For this review, take the finished solid that the model builds, in its own axes (mm). A direction names the side the tool comes from. Coordinates: 2 decimals unless noted, no trailing zeros. Loops run counter-clockwise (first coordinate to the right, second up) from the corner with the lowest first, then second, coordinate; pieces in that order, holes last.
1. Take a section at B-B, the plane z = 0. State the section outline as (x, y) points.
2. Machinability: for faces 1 (the face through (8.8, -1.6, -2.3)), 2 (the face through (10, 0, -2.05)), 3 (the face through (19, 0, 0)), which of the approach directions +Z, -Z, +X, -X, +Y, -Y give a long, thin tool a straight path to every point of the face, cutting with its end or side? Answer none if there is none.
3. Clearance check with a flat-ended pin moving along its axis: P1, Ø5, axis at x = 7, z = 4, coming from the -Y side. State where the tip first meets the part, or that it passes through.
4. To check wall thickness, follow probe 1 along Z at (x, y) = (12.25, 1.15); probe 2 along Y at (x, z) = (7, -2.25); probe 3 along Y at (x, z) = (1, 3.5). State the ranges of each line that lie inside material, in increasing order.
5. Take a section at A-A, the plane x = 11.75. State the section outline as (y, z) points, then the cut area to 3 significant figures.
6. Take a section at C-C, the plane y = 1.55. State the section outline as (x, z) points, then the cut area to 3 significant figures.
7. Take a section at D-D, the plane z = -3. State the section outline as (x, y) points.
```python
from build123d import *

# Parameters (mm, degrees)
SKETCH1_W           = 19
SKETCH1_H           = 10
BOSS_EXTRUDE1_DEPTH = 2
CHAMFER2_SIZE       = 1
SKETCH2_W           = 17.6
SKETCH2_H           = 10
CUT_EXTRUDE4_DEPTH  = 0.4
CUT_EXTRUDE5_DEPTH  = 21.049937656
CHAMFER4_SIZE       = 3.5
CHAMFER4_SIZE2      = 2.450726384
CHAMFER5_SIZE       = 0.25


with BuildPart() as part:
    # Sketch1 → Boss-Extrude1 (new, symmetric)
    with BuildSketch(Plane(origin=(0, 0, 0), x_dir=(1, 0, 0), z_dir=(0, 1, 0))):
        with Locations((9.5, 0)):
            Rectangle(SKETCH1_W, SKETCH1_H)
        with BuildLine():
            Line((8.5, 2.05), (12.5, 2.05))
            ThreePointArc((12.5, 2.05), (14.55, 0), (12.5, -2.05))
            Line((12.5, -2.05), (8.5, -2.05))
            ThreePointArc((8.5, -2.05), (6.45, 0), (8.5, 2.05))
        make_face(mode=Mode.SUBTRACT)
    extrude(amount=BOSS_EXTRUDE1_DEPTH, both=True)

    # Chamfer2
    chamfer2_edges = [part.edges().sort_by_distance(p)[0] for p in [
        (19, 0, -5),
        (19, 0, 5),
    ]]
    chamfer(chamfer2_edges, length=CHAMFER2_SIZE)

    # Sketch2 → Cut-Extrude4 (cut)
    with BuildSketch(Plane(origin=(0, -2, 0), x_dir=(1, 0, 0), z_dir=(0, 1, 0))):
        with Locations((8.8, 0)):
            Rectangle(SKETCH2_W, SKETCH2_H)
    extrude(amount=CUT_EXTRUDE4_DEPTH, mode=Mode.SUBTRACT)

    # Sketch5 → Cut-Extrude5 (cut, through all)
    with BuildSketch(Plane(origin=(0, 2, 0), x_dir=(1, 0, 0), z_dir=(0, 1, 0))):
        Polygon((0, 4), (3.732050808, 5), (0, 5), align=None)
        Polygon((0, -4), (0, -5), (3.732050808, -5), align=None)
    extrude(amount=-CUT_EXTRUDE5_DEPTH, mode=Mode.SUBTRACT)

    # Chamfer4
    chamfer4_edges = [part.edges().sort_by_distance(p)[0] for p in [
        (0, 2, 0),
    ]]
    chamfer4_side = [part.faces().sort_by_distance(p)[0] for p in [
        (1.921596209, 2, -4.29260693),
    ]]
    chamfer(chamfer4_edges, length=CHAMFER4_SIZE, length2=CHAMFER4_SIZE2, reference=chamfer4_side[0])

    # Chamfer5
    chamfer5_edges = [part.edges().sort_by_distance(p)[0] for p in [
        (0, -1.6, 0),
    ]]
    chamfer(chamfer5_edges, length=CHAMFER5_SIZE)


solid = part.part
```
Results list:
1. outline: (0, -1.35) - (0.25, -1.6) - (6.45, -1.6) - (6.45, 2) - (3.5, 2) - (0, -0.45) - close; (14.55, -1.6) - (17.6, -1.6) - (17.6, -2) - (19, -2) - (19, 2) - (14.55, 2) - close
2. face 1: +Z, -Z, -X, -Y
2. face 2: +Y, -Y
2. face 3: +Z, -Z, +X, +Y, -Y
3. P1: stops at y = -1.6
4. probe 1: z = -5 to -2.05, 2.05 to 5
4. probe 2: y = -1.6 to 2
4. probe 3: y = -1.6 to 0.25
5. outline: (-1.6, -5) - (2, -5) - (2, -2.05) - (-1.6, -2.05) - close; (-1.6, 2.05) - (2, 2.05) - (2, 5) - (-1.6, 5) - close
5. area: 21.2 mm2
6. outline: (2.86, -4.77) - (3.73, -5) - (18, -5) - (19, -4) - (19, 4) - (18, 5) - (3.73, 5) - (2.86, 4.77) - close; hole (8.5, -2.05) - (12.5, -2.05) arc R2.05 ccw to (12.5, 2.05) - (8.5, 2.05) arc R2.05 ccw to start
6. area: 131 mm2
7. outline: (0, -1.35) - (0.25, -1.6) - (17.6, -1.6) - (17.6, -2) - (19, -2) - (19, 2) - (3.5, 2) - (0, -0.45) - close
